Could you check a few things on this model? Use its own coordinates, in mm. Face numbers are marked on the shaded views. Give positions to 0.01 mm unless a question says otherwise; leave off trailing zeros. Write each loop counter-clockwise with the first axis right and the second up, starting at its lowest first coordinate (ties: lowest second). Pieces come first, ordered by that corner, then holes. Notation, with made-up numbers: (76.25, 57.5) - (107.25, 57.5) arc R33 ccw to (107.25, 94.5) - close; hole circle Ø3 at (43.25, 23.25). An arc over 180 degrees is marked (long way). Answer in a Markdown table with one row per item.
from build123d import *

# Parameters (mm, degrees)
SKETCH1_W                   = 127.635
SKETCH1_H                   = 127.635
BOSS_EXTRUDE1_DEPTH         = 9.525
SKETCH13_R                  = 93.6625
BOSS_EXTRUDE2_DEPTH         = 9.525
SKETCH5_R                   = 46.355
CUT_EXTRUDE1_DEPTH          = 9.525
SKETCH11_R                  = 1.4351
CUT_EXTRUDE3_DEPTH          = 10.525
CIRPATTERN1_COUNT           = 12
SKETCH12_R                  = 56.41975
CUT_EXTRUDE4_DEPTH          = 1.27
SUPPORT_HOLE_DEPTH          = 6.35
SKETCH16_R                  = 1.27
FRAME_BOLT_HOLE_DEPTH       = 3.175
FRAME_SUPPORT_PATTERN_COUNT = 4


with BuildPart() as part:
    # Sketch1 → Boss-Extrude1 (new body)
    with BuildSketch(Plane(origin=(0, 0, 0), x_dir=(1, 0, 0), z_dir=(0, 1, 0))):
        with Locations((63.8175, 63.8175)):
            Rectangle(SKETCH1_W, SKETCH1_H)
    extrude(amount=BOSS_EXTRUDE1_DEPTH)

    # Sketch13 → Boss-Extrude2 (add)
    with BuildSketch(Plane(origin=(0, 9.525, 0), x_dir=(1, 0, 0), z_dir=(0, 1, 0))):
        with Locations((63.8175, 63.8175)):
            Circle(SKETCH13_R)
    extrude(amount=-BOSS_EXTRUDE2_DEPTH)

    # Sketch5 → Cut-Extrude1 (cut)
    with BuildSketch(Plane(origin=(0, 9.525, 0), x_dir=(1, 0, 0), z_dir=(0, 1, 0))):
        with Locations((63.8175, 63.8175)):
            Circle(SKETCH5_R)
    extrude(amount=-CUT_EXTRUDE1_DEPTH, mode=Mode.SUBTRACT)

    # Sketch11 → Cut-Extrude3 (cut, through all)
    with BuildSketch(Plane(origin=(0, 9.525, 0), x_dir=(1, 0, 0), z_dir=(0, 1, 0))):
        with Locations((63.8175, 115.443)):
            Circle(SKETCH11_R)
    cut_extrude3 = extrude(amount=-CUT_EXTRUDE3_DEPTH, mode=Mode.SUBTRACT)

    # CirPattern1: Cut-Extrude3 ×12 about axis
    cirpattern1_axis = Axis((63.8175, 0, -63.8175), (0, 1, 0))
    for i in range(1, CIRPATTERN1_COUNT):
        add(cut_extrude3.rotate(cirpattern1_axis, i * 360 / CIRPATTERN1_COUNT), mode=Mode.SUBTRACT)

    # Sketch12 → Cut-Extrude4 (cut)
    with BuildSketch(Plane(origin=(0, 9.525, 0), x_dir=(1, 0, 0), z_dir=(0, 1, 0))):
        with Locations((63.8175, 63.8175)):
            Circle(SKETCH12_R)
    extrude(amount=-CUT_EXTRUDE4_DEPTH, mode=Mode.SUBTRACT)

    # Sketch15 → Support hole (cut)
    with BuildSketch(Plane(origin=(0, 9.525, 0), x_dir=(1, 0, 0), z_dir=(0, 1, 0))):
        with BuildLine():
            Line((-20.0025, 63.8175), (-25.0825, 63.8175))
            ThreePointArc((-25.0825, 63.8175), (-22.061832172, 86.794669228), (-13.205102796, 108.21038973))
            Line((-13.205102796, 108.21038973), (-8.745758996, 105.774213931))
            ThreePointArc((-8.745758996, 105.774213931), (-17.139416842, 85.53776739), (-20.0025, 63.8175))
        make_face()
    support_hole = extrude(amount=-SUPPORT_HOLE_DEPTH, mode=Mode.SUBTRACT)

    # Sketch16 → Frame bolt hole (cut)
    with BuildSketch(Plane(origin=(0, 0, 0), x_dir=(-1, 0, 0), z_dir=(0, -1, 0))):
        with Locations((19.592656746, 86.195957311)):
            Circle(SKETCH16_R)
    frame_bolt_hole = extrude(amount=-FRAME_BOLT_HOLE_DEPTH, mode=Mode.SUBTRACT)

    # Frame support pattern: Support hole, Frame bolt hole ×4 about axis
    frame_support_pattern_axis = Axis((63.8175, 0, -63.8175), (0, 1, 0))
    for i in range(1, FRAME_SUPPORT_PATTERN_COUNT):
        add(support_hole.rotate(frame_support_pattern_axis, i * 360 / FRAME_SUPPORT_PATTERN_COUNT), mode=Mode.SUBTRACT)
        add(frame_bolt_hole.rotate(frame_support_pattern_axis, i * 360 / FRAME_SUPPORT_PATTERN_COUNT), mode=Mode.SUBTRACT)


solid = part.part
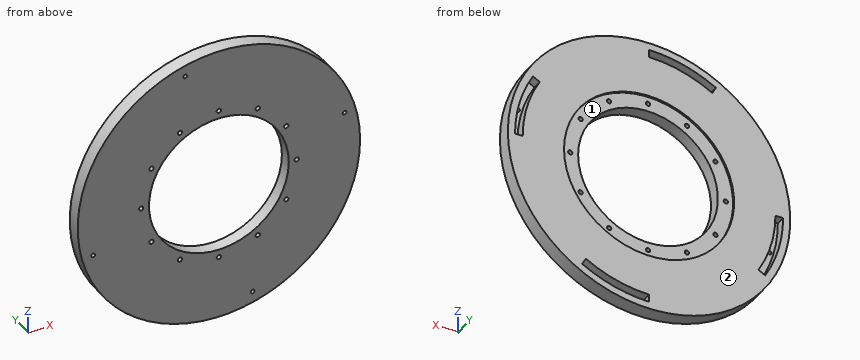
1) If I drill on line 1 (X direction, y = 1.75, z = -63); line 2 (Z direction, x = 74, y = 3.5); line 3 (Z direction, x = 30, y = 5.75), over which ranges is the centre line in solid material (lowest first)?
Check values:
| item | result |
|---|---|
| line 1 | x = -29.84 to 11.01, 13.37 to 17.47, 110.17 to 114.26, 116.62 to 157.48 |
| line 2 | z = -156.92 to -152.13, -147.02 to -109.04, -18.59 to 29.29 |
| line 3 | z = -151.16 to -95.52, -32.11 to 12.88, 18.4 to 23.53 |
2) Will these pins go through, and if not, where does the flat tip stop? P1, Ø5.5, axis at x = 151, y = 7, coming from the +Z side; P2, Ø3, axis at x = -19.59, z = -86.2, coming from the +Y side (3 decimals); P3, Ø2.5, axis at y = 7, z = -150, coming from the +X side.
Check values:
| item | result |
|---|---|
| P1 | stops at z = -23.27 |
| P2 | stops at y = 3.175 |
| P3 | stops at x = 103.3 |
3) Imagine slicing it at D-D (x = 25.5). List the corners of the cut face in (y, z) for me (3 decimals), then the cut area to 3 significant figures.
Check values:
| item | result |
|---|---|
| outline | (0, -149.283) - (9.525, -149.283) - (9.525, -105.23) - (8.255, -105.23) - (8.255, -89.905) - (0, -89.905) - close; (0, -37.73) - (8.255, -37.73) - (8.255, -22.405) - (9.525, -22.405) - (9.525, 10.732) - (3.175, 10.732) - (3.175, 16.401) - (9.525, 16.401) - (9.525, 21.648) - (0, 21.648) - close |
| area | 1,060 mm2 |
4) Imagine slicing it at C-C (z = 16). List the corners of the cut face in (x, y) for me (3 decimals).
Check values:
| item | result |
|---|---|
| outline | (14.809, 0) - (112.826, 0) - (112.826, 9.525) - (38.225, 9.525) - (38.225, 3.175) - (24.672, 3.175) - (24.672, 9.525) - (14.809, 9.525) - close |
5) Imagine slicing it at A-A (x = 94). List the corners of the cut face in (y, z) for me (3 decimals), then the cut area to 3 significant figures.
Check values:
| item | result |
|---|---|
| outline | (0, -152.484) - (9.525, -152.484) - (9.525, -147.437) - (3.175, -147.437) - (3.175, -142.015) - (9.525, -142.015) - (9.525, -111.485) - (8.255, -111.485) - (8.255, -99) - (0, -99) - close; (0, -28.635) - (8.255, -28.635) - (8.255, -16.15) - (9.525, -16.15) - (9.525, 24.849) - (0, 24.849) - close |
| area | 953 mm2 |
6) We'd pull the mould along Z, two halves only. Please class the marked faces 1 and 2: +Z half, -Z half, draft (parallel to the pull), parting line (faces both ways), or undercut.
Check values:
| item | result |
|---|---|
| face 1 | undercut |
| face 2 | draft |
7) Imagine slicing it at B-B (y = 5.75). State how many separate pieces and enclosed holes the cut face has, then the cut area to 3 significant figures.
Check values:
| item | result |
|---|---|
| separate pieces | 1 |
| enclosed holes | 17 |
| area | 19,800 mm2 |
